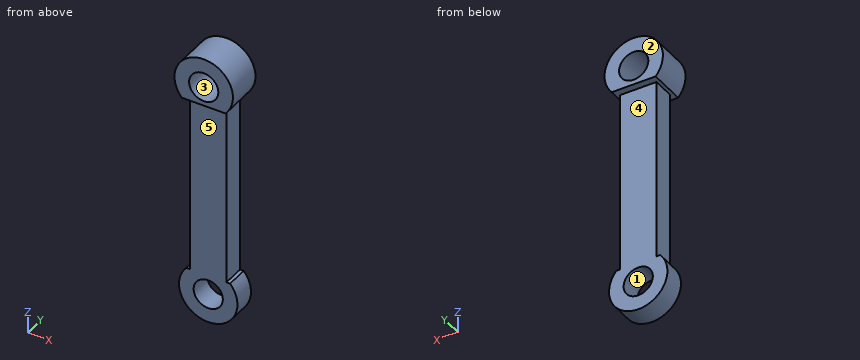
```python
from build123d import *

# Parameters (mm, degrees)
SKETCH1_R           = 2
BOSS_EXTRUDE2_DEPTH = 1.5
SKETCH2_R           = 2
BOSS_EXTRUDE3_DEPTH = 2.5


with BuildPart() as part:
    # Sketch1 → Boss-Extrude2 (new body, symmetric)
    with BuildSketch(Plane(origin=(0, 0, 0), x_dir=(1, 0, 0), z_dir=(0, 1, 0))):
        with BuildLine():
            Line((2.5, 12.499999806), (3, 12.499999806))
            ThreePointArc((3, 12.499999806), (0, 19.145751117), (-3, 12.499999806))
            Line((-3, 12.499999806), (-2.5, 12.499999806))
            Line((-2.5, 12.499999806), (-2.5, -12.499999806))
            Line((-2.5, -12.499999806), (2.5, -12.499999806))
            Line((2.5, -12.499999806), (2.5, 12.499999806))
        make_face()
        with Locations((0, 15.145751117)):
            Circle(SKETCH1_R, mode=Mode.SUBTRACT)
    extrude(amount=BOSS_EXTRUDE2_DEPTH, both=True)

    # Sketch2 → Boss-Extrude3 (add, symmetric)
    with BuildSketch(Plane(origin=(0, 0, 0), x_dir=(1, 0, 0), z_dir=(0, 1, 0))):
        with BuildLine():
            Line((-3, -12.499999806), (3, -12.499999806))
            ThreePointArc((3, -12.499999806), (0, -19.145751117), (-3, -12.499999806))
        make_face()
        with Locations((0, -15.145751117)):
            Circle(SKETCH2_R, mode=Mode.SUBTRACT)
    extrude(amount=BOSS_EXTRUDE3_DEPTH, both=True)


solid = part.part
```
Input: part model. Units: mm. Frame: model coordinates. Face numbers are marked on the shaded views. A direction names the side the tool comes from. Coordinates: 2 decimals unless noted, no trailing zeros. Write each loop counter-clockwise with the first axis right and the second up, starting at its lowest first coordinate (ties: lowest second). Pieces come first, ordered by that corner, then holes. Notation, with made-up numbers: (43, 24) - (77, 24) arc R15 ccw to (77, 49) - close; hole circle Ø9 at (50.5, 49.25). An arc over 180 degrees is marked (long way). Put each result on its own line as item: value. Start each with the question number.
1) Mould query, pull axis Z, two halves, no side actions, for the marked faces 1 and 2. Classes: pulls with the +Z half, pulls with the -Z half, needs draft (parallel to the pull), parting line crosses it, or undercut.
2) Reachability of the marked faces 3, 4 and 5 from +Z, -Z, +X, -X, +Y, -Y: full face, straight path, thin tool, end or side. Return the list, or none.
3) Contact query for flat-ended pins moving along their axis: pin 1 (2.5 mm diameter, centred on x = 2, z = 4, fed in from -Y); pin 2 (1 mm diameter, centred on y = -1, z = 0.5, fed in from -X); pin 3 (2.5 mm diameter, centred on x = 1.5, z = -1, fed in from +Y). Output: stop coordinate, or through.
4) Cut plane B-B (z = 16). Return the cut outline in (x, y).
5) Ray query, L1, parallel to Z at x = 0, y = -0.65; L2, parallel to X at y = -0.3, z = -15; L3, parallel to Z at x = -0.5, y = -0.1. Return the intervals inside material, ascending.
6) Cut plane D-D (z = -2.5). Return the cut outline in (x, y).
7) Cut plane A-A (x = 0). Return the cut outline in (y, z), plus the area to 3 significant figures.
8) Cut plane C-C (y = -1). Return the cut outline in (x, z), plus the area to 3 significant figures.
Resolved:
1. face 1: undercut
1. face 2: needs draft
2. face 3: +Y, -Y
2. face 4: -Z, +X, -X, +Y
2. face 5: -Z, +X, -X, -Y
3. pin 1: stops at y = -1.5
3. pin 2: stops at x = -2.5
3. pin 3: stops at y = 1.5
4. outline: (-3.91, -2.5) - (-1.81, -2.5) - (-1.81, 2.5) - (-3.91, 2.5) - close; (1.81, -2.5) - (3.91, -2.5) - (3.91, 2.5) - (1.81, 2.5) - close
5. L1: z = -19.15 to -17.15, -13.15 to 13.15, 17.15 to 19.15
5. L2: x = -4 to -1.99, 1.99 to 4
5. L3: z = -19.11 to -17.08, -13.21 to 13.21, 17.08 to 19.11
6. outline: (-2.5, -1.5) - (2.5, -1.5) - (2.5, 1.5) - (-2.5, 1.5) - close
7. outline: (-2.5, 12.5) - (-1.5, 12.5) - (-1.5, -13.15) - (1.5, -13.15) - (1.5, 12.5) - (2.5, 12.5) - (2.5, 13.15) - (-2.5, 13.15) - close; (-2.5, 17.15) - (2.5, 17.15) - (2.5, 19.15) - (-2.5, 19.15) - close; (-1.5, -19.15) - (1.5, -19.15) - (1.5, -17.15) - (-1.5, -17.15) - close
7. area: 96.2 mm2
8. outline: (-3, -12.5) arc R4 ccw (long way) to (3, -12.5) - (2.5, -12.5) - (2.5, 12.5) - (3, 12.5) arc R4 ccw (long way) to (-3, 12.5) - (-2.5, 12.5) - (-2.5, -12.5) - close; hole circle Ø4 at (0, -15.15); hole circle Ø4 at (0, 15.15)
8. area: 189 mm2
